```python
from build123d import *

# Parameters (mm, degrees)
F0_W     = 152.390406
F0_H     = 47.625
F1_DEPTH = 57.15
F3_DEPTH = 57.15
F5_DEPTH = 76.2
F6_DEPTH = 127
F8_DEPTH = 50.8


with BuildPart() as f1:
    # F0 (on Front) → F1 (new body)
    with BuildSketch(Plane.XZ):
        with Locations((76.195203, 23.8125)):
            Rectangle(F0_W, F0_H)
    extrude(amount=F1_DEPTH)

    # F2 (on face) → F3 (cut)
    with BuildSketch(Plane.XZ.offset(57.15)):
        Polygon((152.390406, 0), (152.390406, 47.625), (123.815406, 0), align=None)
    extrude(amount=-F3_DEPTH, mode=Mode.SUBTRACT)

    # F4 (on face) → F5 (join)
    with BuildSketch(Plane.XY.offset(47.625)):
        Polygon((0, 0), (152.390406, -28.575), (152.390406, 0), align=None)
    extrude(amount=F5_DEPTH)

    # F5_face (on face) → F6 (cut)
    with BuildSketch(Plane(origin=(101.593604, -9.525, 123.825), x_dir=(1, 0, 0), z_dir=(0, 0, 1))):
        Polygon((-101.593604, 9.525), (50.796802, -19.05), (50.796802, 9.525), align=None)
    extrude(amount=-F6_DEPTH, mode=Mode.SUBTRACT)

    # F7 (on face) → F8 (cut)
    with BuildSketch(Plane.XY.offset(47.625)):
        Polygon((152.390406, -57.15), (152.390406, -28.575), (0, -57.15), align=None)
    extrude(amount=-F8_DEPTH, mode=Mode.SUBTRACT)


solid = f1.part
```
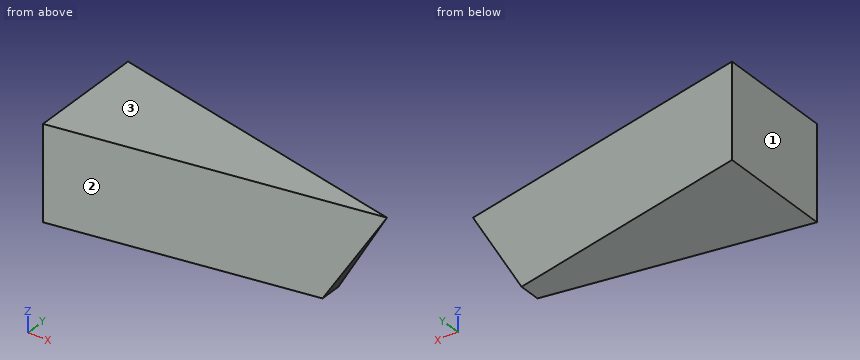
The model under review builds one solid part; all positions refer to its coordinate system, in mm. Face numbers are marked on the shaded views. Coordinates: 2 decimals unless noted, no trailing zeros. Write each loop counter-clockwise with the first axis right and the second up, starting at its lowest first coordinate (ties: lowest second). Pieces come first, ordered by that corner, then holes.
1) Clearance check with flat-ended pins moving along their axes: pin 1 Ø5 at (x, y) = (105.5, -41) entering from -Z; pin 2 Ø5 at (x, z) = (102.5, 10.5) entering from +Y; pin 3 Ø1 at (x, z) = (117.5, 28.5) entering from -Y. State where each tip first meets the part, or that it passes through.
2) We need section A-A on x = 73. State the section outline as (y, z) points (3 decimals).
3) We need section B-B on z = 24. State the section outline as (x, y) points.
4) The part is to be moulded in two halves that separate along X. For the marked faces 1, 2 and 3, say which applies: pulls with the +X half, pulls with the -X half, needs draft (parallel to the pull), parting line crosses it, or undercut.
5) To check wall thickness, follow probe 1 along X at (y, z) = (-29, 27); probe 2 along Y at (x, z) = (123.5, 13); probe 3 along Y at (x, z) = (31.5, 18). State the ranges of each line that lie inside material, in increasing order.
Answer list:
1. pin 1: passes through
1. pin 2: stops at y = -18.75
1. pin 3: stops at y = -35.21
2. outline: (-43.462, 0) - (-13.688, 0) - (-13.688, 47.625) - (-43.462, 47.625) - close
3. outline: (0, -57.15) - (138.22, -31.23) - (138.22, -25.92) - (0, 0) - close
4. face 1: pulls with the -X half
4. face 2: pulls with the +X half
4. face 3: needs draft
5. probe 1: x = 0 to 140.02
5. probe 2: y = -33.99 to -23.16
5. probe 3: y = -51.24 to -5.91
